from build123d import *

# Parameters (mm, degrees)
SKETCH_1_W           = 270
SKETCH_1_H           = 370
SKETCH_1_W_2         = 250
SKETCH_1_H_2         = 350
EXTRUDE_2_DEPTH      = 45
SKETCH_4_W           = 250
SKETCH_4_H           = 350
SKETCH_4_W_2         = 222
SKETCH_4_H_2         = 322
EXTRUDE_3_DEPTH      = 5
SKETCH_9_W           = 246
SKETCH_9_H           = 346
SKETCH_9_W_2         = 226
SKETCH_9_H_2         = 326
CUT_EXTRUDE_3_DEPTH  = 2.5
SKETCH_12_R          = 1.6
CUT_EXTRUDE_5_DEPTH  = 109.5
FILLET_1_R           = 5
SKETCH_13_W          = 250
SKETCH_13_H          = 350
SKETCH_13_W_2        = 222
SKETCH_13_H_2        = 322
EXTRUDE_4_DEPTH      = 33.5
CUT_EXTRUDE_START    = -126.5
SKETCH_14_R          = 1.6
CUT_EXTRUDE_10_DEPTH = 126.5
CUT_EXTRUDE_11_DEPTH = 46
CUT_EXTRUDE_13_DEPTH = 2.5
SKETCH_17_R          = 1.6
CUT_EXTRUDE_14_DEPTH = 75.5


with BuildPart() as part:
    # 草图1 → 凸台-拉伸2 (new body)
    with BuildSketch(Plane(origin=(0, 0, 0), x_dir=(1, 0, 0), z_dir=(0, 1, 0))):
        with Locations((125, 175)):
            Rectangle(SKETCH_1_W, SKETCH_1_H)
        with Locations((125, 175)):
            Rectangle(SKETCH_1_W_2, SKETCH_1_H_2, mode=Mode.SUBTRACT)
    extrude(amount=EXTRUDE_2_DEPTH)

    # 草图4 → 凸台-拉伸3 (add)
    with BuildSketch(Plane(origin=(0, 38.5, 0), x_dir=(1, 0, 0), z_dir=(0, 1, 0))):
        with Locations((125, 175)):
            Rectangle(SKETCH_4_W, SKETCH_4_H)
        with Locations((125, 175)):
            Rectangle(SKETCH_4_W_2, SKETCH_4_H_2, mode=Mode.SUBTRACT)
    extrude(amount=-EXTRUDE_3_DEPTH)

    # 草图9 → 切除-拉伸3 (cut)
    with BuildSketch(Plane(origin=(0, 38.5, 0), x_dir=(1, 0, 0), z_dir=(0, 1, 0))):
        with Locations((125, 175)):
            Rectangle(SKETCH_9_W, SKETCH_9_H)
        with Locations((125, 175)):
            Rectangle(SKETCH_9_W_2, SKETCH_9_H_2, mode=Mode.SUBTRACT)
    extrude(amount=-CUT_EXTRUDE_3_DEPTH, mode=Mode.SUBTRACT)

    # 草图12 → 切除-拉伸5 (cut)
    with BuildSketch(Plane(origin=(0, 45, 0), x_dir=(1, 0, 0), z_dir=(0, 1, 0))):
        with Locations(Location((-3.535533906, -3.535533906, 0), (0, 0, 270))):
            Circle(SKETCH_12_R)
        with BuildLine():
            ThreePointArc((-4.666904756, 354.666904756), (-4.666904756, 352.404163056), (-2.404163056, 352.404163056))
            Line((-2.404163056, 352.404163056), (-4.666904756, 354.666904756))
        make_face()
        with BuildLine():
            Line((-4.666904756, 354.666904756), (-2.404163056, 352.404163056))
            ThreePointArc((-2.404163056, 352.404163056), (-2.057326654, 352.923240414), (-1.935533906, 353.535533906))
            ThreePointArc((-1.935533906, 353.535533906), (-2.923240414, 355.013741158), (-4.666904756, 354.666904756))
        make_face()
        with Locations(Location((253.535533906, 353.535533906, 0), (0, 0, 270))):
            Circle(SKETCH_12_R)
        with Locations(Location((253.535533906, -3.535533906, 0), (0, 0, 270))):
            Circle(SKETCH_12_R)
    extrude(amount=-CUT_EXTRUDE_5_DEPTH, mode=Mode.SUBTRACT)

    # 圆角1
    fillet_1_edges = [part.edges().sort_by_distance(p)[0] for p in [
        (-10, 22.5, 10),
        (-10, 22.5, -360),
        (260, 22.5, -360),
        (260, 22.5, 10),
    ]]
    fillet(fillet_1_edges, radius=FILLET_1_R)

    # 草图13 → 凸台-拉伸4 (add)
    with BuildSketch(Plane.XZ.offset(-33.5)):
        with Locations((125, -175)):
            Rectangle(SKETCH_13_W, SKETCH_13_H)
        with Locations((125, -175)):
            Rectangle(SKETCH_13_W_2, SKETCH_13_H_2, mode=Mode.SUBTRACT)
    extrude(amount=EXTRUDE_4_DEPTH)

    # 草图14 → 切除-拉伸10 (cut)
    # profile 1 of 10: a face of its own
    with BuildSketch(Plane.XZ.offset(CUT_EXTRUDE_START)):
        with BuildLine():
            Line((14, -175), (14, -14))
            Line((14, -14), (14, -6))
            Line((14, -6), (14, 2))
            Line((14, 2), (14, 10))
            Line((14, 10), (-5, 10))
            ThreePointArc((-5, 10), (-8.535533906, 8.535533906), (-10, 5))
            Line((-10, 5), (-10, -175))
            Line((-10, -175), (-2, -175))
            Line((-2, -175), (6, -175))
            Line((6, -175), (14, -175))
        make_face()
        with Locations((-3.535533906, 3.535533906)):
            Circle(SKETCH_14_R, mode=Mode.SUBTRACT)
    # profile 2 of 10: a face of its own
    with BuildSketch(Plane.XZ.offset(CUT_EXTRUDE_START)):
        Polygon((9.5, -181.062177826), (6, -175), (-2, -175), (-5.5, -181.062177826), align=None)
    # profile 3 of 10: a face of its own
    with BuildSketch(Plane.XZ.offset(CUT_EXTRUDE_START)):
        with Locations((-3.535533906, 3.535533906)):
            Circle(SKETCH_14_R)
    # profile 4 of 10: a face of its own
    with BuildSketch(Plane.XZ.offset(CUT_EXTRUDE_START)):
        Polygon((14, -6), (14, -14), (125, -14), (125, 10), (14, 10), (14, 2), (19.975575286, 5.45), (19.975575286, -9.45), align=None)
    # profile 5 of 10: a face of its own
    with BuildSketch(Plane.XZ.offset(CUT_EXTRUDE_START)):
        Polygon((14, 2), (14, -6), (19.975575286, -9.45), (19.975575286, 5.45), align=None)
    # profile 6 of 10: a face of its own
    with BuildSketch(Plane.XZ.offset(CUT_EXTRUDE_START)):
        Polygon((125, 10), (125, -14), (236, -14), (236, -6), (230.024424714, -9.45), (230.024424714, 5.45), (236, 2), (236, 10), align=None)
    # profile 7 of 10: a face of its own
    with BuildSketch(Plane.XZ.offset(CUT_EXTRUDE_START)):
        Polygon((230.024424714, -9.45), (236, -6), (236, 2), (230.024424714, 5.45), align=None)
    # profile 8 of 10: a face of its own
    with BuildSketch(Plane.XZ.offset(CUT_EXTRUDE_START)):
        with BuildLine():
            Line((236, -336), (14, -336))
            Line((14, -336), (14, -344))
            Line((14, -344), (19.975575286, -340.55))
            Line((19.975575286, -340.55), (19.975575286, -355.45))
            Line((19.975575286, -355.45), (14, -352))
            Line((14, -352), (14, -360))
            Line((14, -360), (255, -360))
            ThreePointArc((255, -360), (258.535533906, -358.535533906), (260, -355))
            Line((260, -355), (260, 5))
            ThreePointArc((260, 5), (258.535533906, 8.535533906), (255, 10))
            Line((255, 10), (236, 10))
            Line((236, 10), (236, 2))
            Line((236, 2), (236, -6))
            Line((236, -6), (236, -14))
            Line((236, -14), (236, -336))
        make_face()
        with Locations((253.535533906, -353.535533906)):
            Circle(SKETCH_14_R, mode=Mode.SUBTRACT)
        with Locations((253.535533906, 3.535533906)):
            Circle(SKETCH_14_R, mode=Mode.SUBTRACT)
    # profile 9 of 10: a face of its own
    with BuildSketch(Plane.XZ.offset(CUT_EXTRUDE_START)):
        with Locations((253.535533906, 3.535533906)):
            Circle(SKETCH_14_R)
    # profile 10 of 10: a face of its own
    with BuildSketch(Plane.XZ.offset(CUT_EXTRUDE_START)):
        with Locations((253.535533906, -353.535533906)):
            Circle(SKETCH_14_R)
    extrude(amount=CUT_EXTRUDE_10_DEPTH, mode=Mode.SUBTRACT)

    # 草图15 → 切除-拉伸11 (cut)
    with BuildSketch(Plane(origin=(0, 45, 0), x_dir=(1, 0, 0), z_dir=(0, 1, 0))):
        with BuildLine():
            Line((-5, 358), (12, 358))
            Line((12, 358), (14, 358))
            Line((14, 358), (14, 360))
            Line((14, 360), (-5, 360))
            ThreePointArc((-5, 360), (-8.535533906, 358.535533906), (-10, 355))
            Line((-10, 355), (-10, 175))
            Line((-10, 175), (-8, 175))
            Line((-8, 175), (-8, 177))
            Line((-8, 177), (-8, 355))
            ThreePointArc((-8, 355), (-7.121320344, 357.121320344), (-5, 358))
        make_face()
    extrude(amount=-CUT_EXTRUDE_11_DEPTH, mode=Mode.SUBTRACT)

    # 草图16 → 切除-拉伸13 (cut)
    with BuildSketch(Plane(origin=(0, 38.5, 0), x_dir=(1, 0, 0), z_dir=(0, 1, 0))):
        Polygon((19.975575286, 348), (19.975575286, 350), (0, 350), (0, 181.062177826), (2, 181.062177826), (2, 348), align=None)
    extrude(amount=-CUT_EXTRUDE_13_DEPTH, mode=Mode.SUBTRACT)

    # 草图17 → 切除-拉伸14 (cut)
    with BuildSketch(Plane(origin=(0, 45, 0), x_dir=(1, 0, 0), z_dir=(0, 1, 0))):
        with Locations(Location((-3.535533906, 273.535533906, 0), (0, 0, 270))):
            Circle(SKETCH_17_R)
    extrude(amount=-CUT_EXTRUDE_14_DEPTH, mode=Mode.SUBTRACT)


solid = part.part
Here's how the part is built. I have some questions about the finished solid (model axes, mm). A direction names the side the tool comes from. Round coordinates to 2 decimals unless told otherwise and drop trailing zeros. Write each loop counter-clockwise with the first axis right and the second up, starting at its lowest first coordinate (ties: lowest second). Pieces come first, ordered by that corner, then holes. Notation, with made-up numbers: (-8, -30.5) -> (18, -30.5) arc R27 cw to (18, -6.5) -> close; hole circle Ø7 at (-3, 24.5). An arc over 180 degrees is marked (long way). One line per item, written item: value.
1) For faces 1 (the face through (-7.14, 22.82, -357.1)), 2 (the face through (7.774, 18.252, -178.074)), 3 (the face through (0, 41, -267)), which set-ups out of +Z, -Z, +X, -X, +Y, -Y let a thin tool reach every point of the face, with its end or its side?
Filled sheet:
face 1: -Z, -X, +Y, -Y
face 2: +Y, -Y
face 3: +Z, +Y
2) If I drill on line 1 (Z direction, x = 13, y = 38); line 2 (X direction, y = 37.5, z = -277.5); line 3 (Z direction, x = -4.25, y = 22.5), over which ranges is the centre line in solid material (lowest first)? Write a range as [from, to].
Filled sheet:
line 1: z = [-358, -350], [-338, -175]
line 2: x = [-8, 0], [12, 14]
line 3: z = [-358, -354.97], [-352.1, -274.97], [-272.1, -181.06], [-178.9, -175]
3) Suppose I cut it at D-D on z = -347. List the corners of the cut face in (x, y) for me, plus the area to 3 significant figures.
Filled sheet:
outline: (-8, 0) -> (19.98, 0) -> (19.98, 36) -> (0, 36) -> (0, 45) -> (-8, 45) -> close
area: 1,080 mm2
4) I'm going to push flat-ended pins straight in: pin 1 Ø11.5 at (y, z) = (23.5, -289) entering from +X; pin 2 Ø3 at (x, z) = (4, -288) entering from +Y; pin 3 Ø3 at (x, z) = (-3.54, -273.54) entering from -Y; pin 4 Ø2.5 at (x, y) = (9, 39.5) entering from +Z. Where does each tip first touch, or does it pass through?
Filled sheet:
pin 1: stops at x = 14
pin 2: stops at y = 36
pin 3: passes through
pin 4: stops at z = -350
5) We'd pull the mould along X, two halves only. Please class faces 4 (the face through (4, 23, -358)), 5 (the face through (5, 36, -264)), 6 (the face through (19.976, 18, -348)), 7 (the face through (2, 18, -181.062)): released by +X, released by -X, zero draft, split by the parting line, or undercut.
Filled sheet:
face 4: zero draft
face 5: undercut
face 6: released by +X
face 7: undercut
6) Suppose I cut it at C-C on y = 20. List the corners of the cut face in (x, z) for me.
Filled sheet:
outline: (-8, -355) arc R3 ccw to (-5, -358) -> (14, -358) -> (14, -352) -> (19.98, -355.45) -> (19.98, -340.55) -> (14, -344) -> (14, -175) -> (6, -175) -> (9.5, -181.06) -> (-5.5, -181.06) -> (-2, -175) -> (-8, -175) -> close; hole circle Ø3.2 at (-3.54, -353.54); hole circle Ø3.2 at (-3.54, -273.54)
7) Suppose I cut it at B-B on x = 4.25. List the corners of the cut face in (y, z) for me.
Filled sheet:
outline: (0, -358) -> (45, -358) -> (45, -350) -> (36, -350) -> (36, -181.06) -> (0, -181.06) -> close
8) Suppose I cut it at A-A on z = -301. List the corners of the cut face in (x, y) for me, plus the area to 3 significant figures.
Filled sheet:
outline: (-8, 0) -> (14, 0) -> (14, 38.5) -> (12, 38.5) -> (12, 36) -> (0, 36) -> (0, 45) -> (-8, 45) -> close
area: 869 mm2
